```python
from build123d import *

# Parameters (mm, degrees)
SKETCH1_W                                        = 101.6
SKETCH1_H                                        = 50.8
BOSS_EXTRUDE1_DEPTH                              = 25.4
CBORE_FOR_1_4_SOCKET_HEAD_CAP_SCREW1_D           = 6.7564
CBORE_FOR_1_4_SOCKET_HEAD_CAP_SCREW1_CBORE_D     = 11.1125
CBORE_FOR_1_4_SOCKET_HEAD_CAP_SCREW1_CBORE_DEPTH = 6.35
LPATTERN1_COUNT                                  = 4
LPATTERN1_PITCH                                  = 25.4
F_1_4_CLEARANCE_HOLE1_D                          = 6.7564
LPATTERN2_COUNT                                  = 4
LPATTERN2_PITCH                                  = 25.4
SKETCH7_W                                        = 101.6
SKETCH7_H                                        = 9.525
BOSS_EXTRUDE2_DEPTH                              = 19.05
SKETCH8_W                                        = 50.8
SKETCH8_H                                        = 9.525
CUT_EXTRUDE1_DEPTH                               = 19.05
LPATTERN3_COUNT                                  = 2
LPATTERN3_PITCH                                  = 25.4
LPATTERN4_COPY_1_D                               = 6.7564
LPATTERN4_COPY_2_D                               = 6.7564


with BuildPart() as part:
    # Sketch1 → Boss-Extrude1 (new body)
    with BuildSketch(Plane(origin=(0, 0, 0), x_dir=(1, 0, 0), z_dir=(0, 1, 0))):
        with Locations((50.8, 25.4)):
            Rectangle(SKETCH1_W, SKETCH1_H)
    extrude(amount=BOSS_EXTRUDE1_DEPTH)

    # CBORE for 1/4 Socket Head Cap Screw1 (through all)
    with Locations(Plane(origin=(0, 25.4, 0), x_dir=(-1, 0, 0), z_dir=(0, 1, 0))):
        with Locations((-12.7, -12.7)):
            cbore_for_1_4_socket_head_cap_screw1 = CounterBoreHole(CBORE_FOR_1_4_SOCKET_HEAD_CAP_SCREW1_D / 2, CBORE_FOR_1_4_SOCKET_HEAD_CAP_SCREW1_CBORE_D / 2, CBORE_FOR_1_4_SOCKET_HEAD_CAP_SCREW1_CBORE_DEPTH)

    # LPattern1: CBORE for 1/4 Socket Head Cap Screw1 ×4
    with Locations(*[(i * LPATTERN1_PITCH, 0, 0) for i in range(1, LPATTERN1_COUNT)]):
        add(cbore_for_1_4_socket_head_cap_screw1, mode=Mode.SUBTRACT)

    # 1/4 Clearance Hole1 (through all)
    with Locations(Plane(origin=(0, 25.4, 0), x_dir=(-1, 0, 0), z_dir=(0, 1, 0))):
        with Locations((-12.7, -38.1)):
            f_1_4_clearance_hole1 = Hole(F_1_4_CLEARANCE_HOLE1_D / 2)

    # LPattern2: 1/4 Clearance Hole1 ×4
    with Locations(*[(i * LPATTERN2_PITCH, 0, 0) for i in range(1, LPATTERN2_COUNT)]):
        add(f_1_4_clearance_hole1, mode=Mode.SUBTRACT)

    # Sketch7 → Boss-Extrude2 (add)
    with BuildSketch(Plane(origin=(0, 0, -50.8), x_dir=(-1, 0, 0), z_dir=(0, 0, -1))):
        with Locations((-50.8, 20.6375)):
            Rectangle(SKETCH7_W, SKETCH7_H)
    extrude(amount=BOSS_EXTRUDE2_DEPTH)

    # Sketch8 → Cut-Extrude1 (cut)
    with BuildSketch(Plane(origin=(0, 0, -69.85), x_dir=(-1, 0, 0), z_dir=(0, 0, -1))):
        with Locations((-50.8, 20.6375)):
            Rectangle(SKETCH8_W, SKETCH8_H)
    extrude(amount=-CUT_EXTRUDE1_DEPTH, mode=Mode.SUBTRACT)

    # LPattern3: 1/4 Clearance Hole1 ×2
    with Locations(*[(0, 0, -i * LPATTERN3_PITCH) for i in range(1, LPATTERN3_COUNT)]):
        add(f_1_4_clearance_hole1, mode=Mode.SUBTRACT)

    # LPattern4 copy 1 (through all)
    with Locations(Plane(origin=(76.2, 25.4, -25.4), x_dir=(-1, 0, 0), z_dir=(0, 1, 0))):
        with Locations((-12.7, -38.1)):
            Hole(LPATTERN4_COPY_1_D / 2)

    # LPattern4 copy 2 (through all)
    with Locations(Plane(origin=(76.2, 25.4, 0), x_dir=(-1, 0, 0), z_dir=(0, 1, 0))):
        with Locations((-12.7, -38.1)):
            Hole(LPATTERN4_COPY_2_D / 2)


solid = part.part
```
Input: part model. Units: mm. Frame: model coordinates. A direction names the side the tool comes from. Give positions to 0.01 mm unless a question says otherwise; leave off trailing zeros. Loops run counter-clockwise (first coordinate to the right, second up) from the corner with the lowest first, then second, coordinate; pieces in that order, holes last.
1) Contact query for flat-ended pins moving along their axis: pin 1 (5.5 mm diameter, centred on x = 88.5, z = -10.5, fed in from +Y); pin 2 (3 mm diameter, centred on x = 62.5, y = 12.5, fed in from -Z). Output: stop coordinate, or through.
A:
pin 1: stops at y = 19.05
pin 2: stops at z = -50.8
2) Section query A-A on z = -38.1. Return the cut outline in (x, y), and give its area (3 significant figures).
A:
outline: (0, 0) - (9.32, 0) - (9.32, 25.4) - (0, 25.4) - close; (16.08, 0) - (34.72, 0) - (34.72, 25.4) - (16.08, 25.4) - close; (41.48, 0) - (60.12, 0) - (60.12, 25.4) - (41.48, 25.4) - close; (66.88, 0) - (85.52, 0) - (85.52, 25.4) - (66.88, 25.4) - close; (92.28, 0) - (101.6, 0) - (101.6, 25.4) - (92.28, 25.4) - close
area: 1,890 mm2
3) Mould query, pull axis Z, two halves, no side actions, for faces 4 (the flat face through (50, 13, 0)), 5 (the flat face through (10, 19.05, -15)), 6 (the flat face through (89, 19.05, -16.3)), 7 (the flat face through (89, 15.875, -58)). Classes: released by +Z, released by -Z, zero draft, split by the parting line, or undercut.
A:
face 4: released by +Z
face 5: undercut
face 6: undercut
face 7: zero draft
4) Section query C-C on x = 88.9. Return the cut outline in (y, z) (3 decimals), and give its area (3 significant figures).
A:
outline: (0, -50.8) - (15.875, -50.8) - (15.875, -60.122) - (25.4, -60.122) - (25.4, -41.478) - (0, -41.478) - close; (0, -34.722) - (25.4, -34.722) - (25.4, -18.256) - (19.05, -18.256) - (19.05, -16.078) - (0, -16.078) - close; (0, -9.322) - (19.05, -9.322) - (19.05, -7.144) - (25.4, -7.144) - (25.4, 0) - (0, 0) - close; (15.875, -69.85) - (25.4, -69.85) - (25.4, -66.878) - (15.875, -66.878) - close
area: 1,040 mm2
5) Line query: L1, parallel to Z at x = 12.7, y = 19.5; L2, parallel to Z at x = 12.5, y = 4.25; L3, parallel to Z at x = 65.5, y = 8. Output: solid intervals per line, ascending.
A:
L1: z = -69.85 to -66.88, -60.12 to -41.48, -34.72 to -18.26, -7.14 to 0
L2: z = -50.8 to -41.47, -34.73 to -16.07, -9.33 to 0
L3: z = -50.8 to -40.82, -35.38 to -15.42, -9.98 to 0
6) Section query B-B on y = 20.5. Count the separate pieces of the cut face and the enclosed holes in it, and give its area (3 significant figures).
A:
separate pieces: 1
enclosed holes: 10
area: 5,530 mm2
7) Section query D-D on x = 38.1. Return the cut outline in (y, z), and give its area (3 significant figures).
A:
outline: (0, -50.8) - (25.4, -50.8) - (25.4, -41.48) - (0, -41.48) - close; (0, -34.72) - (25.4, -34.72) - (25.4, -18.26) - (19.05, -18.26) - (19.05, -16.08) - (0, -16.08) - close; (0, -9.32) - (19.05, -9.32) - (19.05, -7.14) - (25.4, -7.14) - (25.4, 0) - (0, 0) - close
area: 919 mm2
8) Reachability of faces 1 (the flat face through (13, 15.875, -58)), 2 (the flat face through (38.2, 19.05, -16.3)), 3 (the flat face through (76.2, 21, -60)) from +Z, -Z, +X, -X, +Y, -Y: full face, straight path, thin tool, end or side. Return the list, or none.
A:
face 1: -Z, +X, -X, -Y
face 2: +Y
face 3: -Z, +Y, -Y
